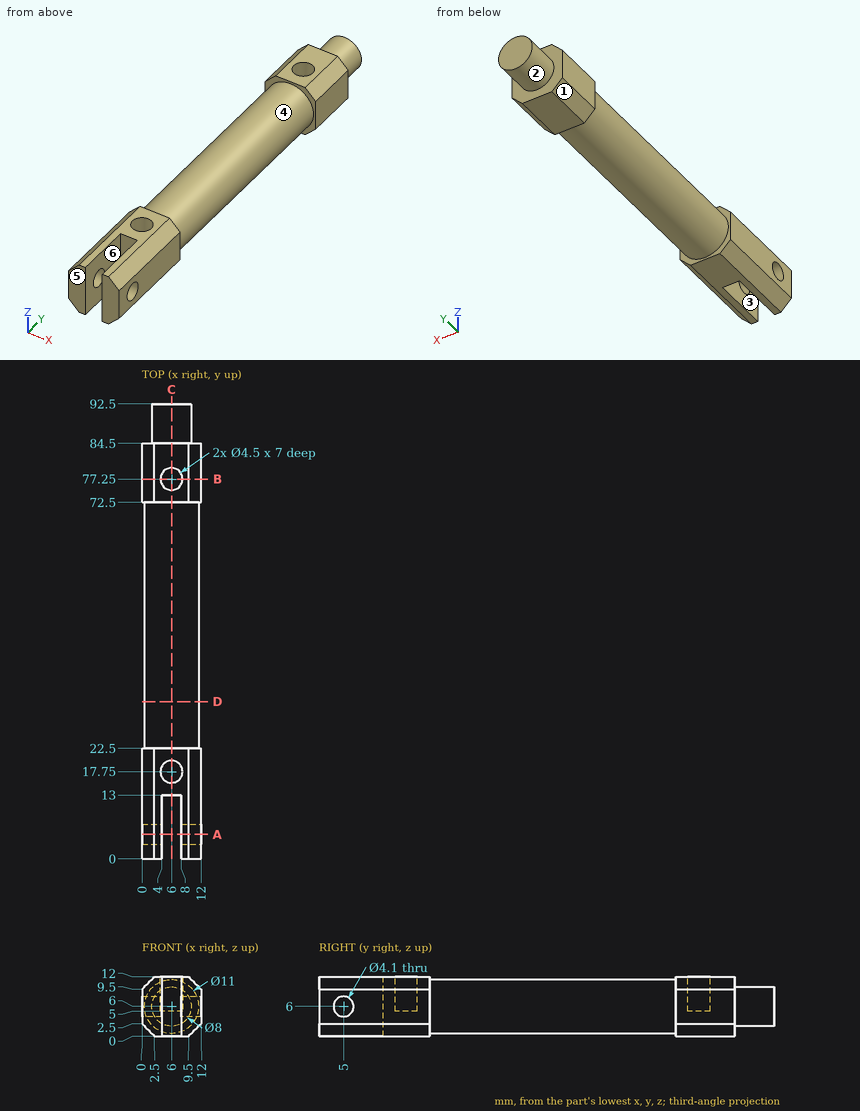
Geometry check sheet. Reference: drawing and pictorial views, mm from the part's lowest x, y, z. A direction names the side the tool comes from. Give positions to 0.01 mm unless a question says otherwise; leave off trailing zeros. Order: outer loops, then holes, each group sorted by start corner. A loop starts at its lowest first (then second) coordinate and runs counter-clockwise, first axis right, second up. Notation, with made-up numbers: M -2,20.5 L 43,20.5 A24 cw 43,58.5 Z; hole C 69,87.5 d4. An arc over 180 degrees is marked long. Return JSON: item names as keys, results as strings. Group by question number.
1) Section check A-A on y = 5. Record the cut outline in (x, z), and give its area (3 significant figures).
2) Section check C-C on x = 6. Record the cut outline in (y, z).
3) Scan lines: line 1 (Y direction, x = 6, z = 8); line 2 (Y direction, x = 2.75, z = 0.5); line 3 (X direction, y = 17.75, z = 7). Record each from-to range of solid material in increasing order.
4) Go/stop test with flat-tipped pins: pin 1 Ø6 at (x, y) = (4, 51.5) entering from +Z; pin 2 Ø6 at (y, z) = (58, 4) entering from +X; pin 3 Ø1.2 at (x, z) = (7, 5) entering from -Y. Record where each tip stops, or that it passes through.
5) Section check B-B on y = 77.25. Record the cut outline in (x, z), and give its area (4 significant figures).
6) Section check D-D on y = 32. Record the cut outline in (x, z), and give its area (3 significant figures).
7) Mould release check, pull along Y, two halves, no side actions. Record for the marked faces 4, 5 and 6: pulls with the +Y half, pulls with the -Y half, needs draft (parallel to the pull), parting line crosses it, or undercut.
8) Access from +Z, -Z, +X, -X, +Y, -Y to the whole of each face (thin tool, end or side, straight path). Record for the marked faces 1, 2 and 3.
Answer block:
{
 "1": {"outline": "M 0,2.5 L 2.5,0 L 4,0 L 4,3.95 L 0,3.95 Z; M 0,8.05 L 4,8.05 L 4,12 L 2.5,12 L 0,9.5 Z; M 8,0 L 9.5,0 L 12,2.5 L 12,3.95 L 8,3.95 Z; M 8,8.05 L 12,8.05 L 12,9.5 L 9.5,12 L 8,12 Z", "area": "50.7 mm^2"},
 "2": {"outline": "M 13,0 L 22.5,0 L 22.5,0.5 L 72.5,0.5 L 72.5,0 L 84.5,0 L 84.5,2 L 92.5,2 L 92.5,10 L 84.5,10 L 84.5,12 L 79.5,12 L 79.5,5 L 75,5 L 75,12 L 72.5,12 L 72.5,11.5 L 22.5,11.5 L 22.5,12 L 20,12 L 20,5 L 15.5,5 L 15.5,12 L 13,12 Z"},
 "3": {"line 1": "y = 13 to 15.5, 20 to 75, 79.5 to 92.5", "line 2": "y = 0 to 22.5, 72.5 to 84.5", "line 3": "x = 0 to 3.75, 8.25 to 12"},
 "4": {"pin 1": "stops at z = 11.5", "pin 2": "stops at x = 11.5", "pin 3": "stops at y = 13"},
 "5": {"outline": "M 0,2.5 L 2.5,0 L 9.5,0 L 12,2.5 L 12,9.5 L 9.5,12 L 8.25,12 L 8.25,5 L 3.75,5 L 3.75,12 L 2.5,12 L 0,9.5 Z", "area": "100.0 mm^2"},
 "6": {"outline": "C 6,6 d11", "area": "95.0 mm^2"},
 "7": {"face 4": "undercut", "face 5": "pulls with the -Y half", "face 6": "needs draft"},
 "8": {"face 1": "-Z, -X, +Y, -Y", "face 2": "+Y", "face 3": "+Z, -Z, -Y"}
}
